Verification items for the finished model (mm, model axes). A direction names the side the tool comes from. Coordinates: 2 decimals unless noted, no trailing zeros. Order: outer loops, then holes, each group sorted by start corner. A loop starts at its lowest first (then second) coordinate and runs counter-clockwise, first axis right, second up. Notation, with made-up numbers: (-24, 42) - (10, 42) arc R24 ccw to (10, 64) - close; hole circle Ø2 at (-38.75, 68). An arc over 180 degrees is marked (long way). Answer as CSV lines item,"result". Start each with the question number.
1. Go/stop test with flat-tipped pins: pin 1 (1.5 mm diameter, centred on y = 5, z = -7.5, fed in from -X); pin 2 (3 mm diameter, centred on x = 7, y = 4.5, fed in from +Z); pin 3 (1.5 mm diameter, centred on x = 8.5, y = 7, fed in from +Z). Record where each tip stops, or that it passes through.
2. Mould release check, pull along X, two halves, no side actions. Record for faces 4 (the cylindrical face through (36.36, 0.44, -1.39)), 5 (the flat face through (9, 5.08, -13)), 6 (the flat face through (0, 0.4, -15.2)), 7 (the flat face through (13.398, 3, -5)): pulls with the +X half, pulls with the -X half, needs draft (parallel to the pull), parting line crosses it, or undercut.
3. Section check B-B (y = 3.5). Record the cut outline in (x, z) (1 decimal), and give its area (3 significant figures).
4. Material ranges on L1, parallel to X at y = 5, z = -7; L2, parallel to Z at x = 7.5, y = 4.75; L3, parallel to Z at x = 25, y = 1.75, recorded low to high. Write a range as [from, to].
5. Set-up check for faces 1 (the flat face through (29.146, 3, -11)), 2 (the flat face through (13.398, 3, -13)), 3 (the flat face through (25, 5.08, -11)): record each of +Z, -Z, +X, -X, +Y, -Y from which the full face is reachable in a straight line by a thin tool's end or side.
6. Section check D-D (z = -4). Record the cut outline in (x, y), and give its area (3 significant figures).
7. Section check C-C (x = 28). Record the cut outline in (y, z).
8. Section check A-A (x = 35.56). Record the cut outline in (y, z), and give its area (3 significant figures).
from build123d import *

# Parameters (mm, degrees)
SKETCH1_W           = 37.4396
SKETCH1_H           = 30.734
SKETCH1_R           = 0.9525
BOSS_EXTRUDE1_DEPTH = 0.889
SKETCH2_R           = 2.032
BOSS_EXTRUDE2_DEPTH = 7.62
SKETCH3_W           = 16.51
SKETCH3_H           = 8.255
SKETCH3_R           = 0.9525
BOSS_EXTRUDE4_DEPTH = 7.62
SKETCH4_W           = 8.001
SKETCH4_H           = 8.001
BOSS_EXTRUDE5_DEPTH = 4.191


with BuildPart() as part:
    # Sketch1 → Boss-Extrude1 (new body)
    with BuildSketch(Plane(origin=(0, 0, 0), x_dir=(1, 0, 0), z_dir=(0, 1, 0))):
        with Locations((18.7198, 15.367)):
            Rectangle(SKETCH1_W, SKETCH1_H)
        with Locations(Location((19.939, 28.702, 0), (0, 0, 270))):
            Circle(SKETCH1_R, mode=Mode.SUBTRACT)
        with Locations(Location((35.56, 1.905, 0), (0, 0, 270))):
            Circle(SKETCH1_R, mode=Mode.SUBTRACT)
        with Locations(Location((1.905, 18.8722, 0), (0, 0, 270))):
            Circle(SKETCH1_R, mode=Mode.SUBTRACT)
    extrude(amount=BOSS_EXTRUDE1_DEPTH)

    # Sketch2 → Boss-Extrude2 (add)
    with BuildSketch(Plane(origin=(0, 0.889, 0), x_dir=(1, 0, 0), z_dir=(0, 1, 0))):
        with Locations(Location((12.065, 20.066, 0), (0, 0, 90))):
            Circle(SKETCH2_R)
        with Locations(Location((18.034, 20.066, 0), (0, 0, 90))):
            Circle(SKETCH2_R)
    extrude(amount=BOSS_EXTRUDE2_DEPTH)

    # Sketch3 → Boss-Extrude4 (add)
    # profile 1 of 3: a face of its own
    with BuildSketch(Plane(origin=(0, 0.889, 0), x_dir=(1, 0, 0), z_dir=(0, 1, 0))):
        with Locations((17.78, 26.6065)):
            Rectangle(SKETCH3_W, SKETCH3_H)
        with Locations(Location((19.939, 28.702, 0), (0, 0, 270))):
            Circle(SKETCH3_R, mode=Mode.SUBTRACT)
    # profile 2 of 3: a face of its own
    with BuildSketch(Plane(origin=(0, 0.889, 0), x_dir=(1, 0, 0), z_dir=(0, 1, 0))):
        with Locations(Location((19.939, 28.702, 0), (0, 0, 270))):
            Circle(SKETCH3_R)
    # profile 3 of 3: a face of its own
    with BuildSketch(Plane(origin=(0, 0.889, 0), x_dir=(1, 0, 0), z_dir=(0, 1, 0))):
        Polygon((6.985, 30.734), (6.985, 18.034), (9.525, 18.034), (9.525, 22.479), (9.525, 30.734), align=None)
    extrude(amount=BOSS_EXTRUDE4_DEPTH)

    # Sketch4 → Boss-Extrude5 (add)
    with BuildSketch(Plane(origin=(0, 0.889, 0), x_dir=(1, 0, 0), z_dir=(0, 1, 0))):
        with Locations((24.765, 10.795)):
            Rectangle(SKETCH4_W, SKETCH4_H)
        with Locations((33.147, 10.795)):
            Rectangle(SKETCH4_W, SKETCH4_H)
        with Locations((9.398, 4.699)):
            Rectangle(SKETCH4_W, SKETCH4_H)
        with Locations((9.398, 13.081)):
            Rectangle(SKETCH4_W, SKETCH4_H)
    extrude(amount=BOSS_EXTRUDE5_DEPTH)


solid = part.part
Evaluation:
1,pin 1,"stops at x = 5.4"
1,pin 2,"stops at z = -0.7"
1,pin 3,"stops at z = -18.03"
2,face 4,"undercut"
2,face 5,"needs draft"
2,face 6,"pulls with the -X half"
2,face 7,"undercut"
3,outline,"(5.4, -17.1) - (13.4, -17.1) - (13.4, -9.1) - (5.4, -9.1) - close; (5.4, -8.7) - (13.4, -8.7) - (13.4, -0.7) - (5.4, -0.7) - close; (7, -30.7) - (26, -30.7) - (26, -22.5) - (9.5, -22.5) - (9.5, -18) - (7, -18) - close; circle Ø4.1 at (12.1, -20.1); circle Ø4.1 at (18, -20.1); (20.8, -14.8) - (28.8, -14.8) - (28.8, -6.8) - (20.8, -6.8) - close; (29.1, -14.8) - (37.1, -14.8) - (37.1, -6.8) - (29.1, -6.8) - close"
3,area,"451 mm²"
4,L1,"x = [5.4, 13.4], [20.76, 28.77], [29.15, 37.15]"
4,L2,"z = [-30.73, -18.03], [-17.08, -9.08], [-8.7, -0.7]"
4,L3,"z = [-30.73, -22.48], [-14.8, -6.79]"
5,face 1,"+Z, -Z, +Y"
5,face 2,"+Z, +Y"
5,face 3,"+Z, +X, -X, +Y"
6,outline,"(0, 0) - (37.44, 0) - (37.44, 0.89) - (13.4, 0.89) - (13.4, 5.08) - (5.4, 5.08) - (5.4, 0.89) - (0, 0.89) - close"
6,area,"66.8 mm²"
7,outline,"(0, -30.73) - (0.89, -30.73) - (0.89, -14.8) - (5.08, -14.8) - (5.08, -6.79) - (0.89, -6.79) - (0.89, 0) - (0, 0) - close"
8,outline,"(0, -30.73) - (0.89, -30.73) - (0.89, -14.8) - (5.08, -14.8) - (5.08, -6.79) - (0.89, -6.79) - (0.89, -2.86) - (0, -2.86) - close; (0, -0.95) - (0.89, -0.95) - (0.89, 0) - (0, 0) - close"
8,area,"59.2 mm²"
